Design review of the part built by this model. Coordinates are the model's own, in mm. Round coordinates to 2 decimals unless told otherwise and drop trailing zeros. Loops run counter-clockwise (first coordinate to the right, second up) from the corner with the lowest first, then second, coordinate; pieces in that order, holes last. Notation, with made-up numbers: M 55.5,-40 L 110.5,-40 A16 ccw 110.5,-21 Z; hole C -37,41.5 d1. An arc over 180 degrees is marked long. Use a Markdown table: item, result.
from build123d import *

# Parameters (mm, degrees)
ESQUISSE1_W              = 160
ESQUISSE1_H              = 210
BOSS_EXTRU_1_DEPTH       = 3
CONG_6_R                 = 2
ESQUISSE4_R              = 1.5
ENL_V_MAT_EXTRU_3_DEPTH  = 4
ESQUISSE6_W              = 45
ESQUISSE6_H              = 70
ENL_V_MAT_EXTRU_5_DEPTH  = 4
ESQUISSE7_R              = 15
ENL_V_MAT_EXTRU_6_DEPTH  = 856
ESQUISSE8_R              = 15
ENL_V_MAT_EXTRU_7_DEPTH  = 856
ESQUISSE9_R              = 7.5
ENL_V_MAT_EXTRU_8_DEPTH  = 856
ESQUISSE10_R             = 7.5
ENL_V_MAT_EXTRU_13_DEPTH = 856
ESQUISSE12_W             = 30
ESQUISSE12_H             = 15
ENL_V_MAT_EXTRU_14_DEPTH = 856
ESQUISSE13_W             = 160
ESQUISSE13_H             = 3
BOSS_EXTRU_2_DEPTH       = 3
ESQUISSE14_W             = 3
ESQUISSE14_H             = 213
BOSS_EXTRU_3_DEPTH       = 3
ESQUISSE15_W             = 3
ESQUISSE15_H             = 70
ENL_V_MAT_EXTRU_15_DEPTH = 4
ESQUISSE18_W             = 3
ESQUISSE18_H             = 213
BOSS_EXTRU_4_DEPTH       = 3
ESQUISSE19_W             = 166
ESQUISSE19_H             = 3
BOSS_EXTRU_5_DEPTH       = 3
ESQUISSE20_W             = 3
ESQUISSE20_H             = 70
ENL_V_MAT_EXTRU_16_DEPTH = 3
ESQUISSE21_R             = 1.5
ENL_V_MAT_EXTRU_17_DEPTH = 3
ESQUISSE22_R             = 1.5
ENL_V_MAT_EXTRU_18_DEPTH = 3
ESQUISSE23_R             = 1.5
ENL_V_MAT_EXTRU_19_DEPTH = 3
CONG_7_R                 = 2
CONG_8_R                 = 2
CONG_9_R                 = 2


with BuildPart() as part:
    # Esquisse1 → Boss.-Extru.1 (new body)
    with BuildSketch(Plane.XY):
        with Locations((-86.269341233, 25.410958904)):
            Rectangle(ESQUISSE1_W, ESQUISSE1_H)
    extrude(amount=BOSS_EXTRU_1_DEPTH)

    # Congé6
    cong_6_edges = [part.edges().sort_by_distance(p)[0] for p in [
        (-166.269341233, 130.410958904, 1.5),
    ]]
    fillet(cong_6_edges, radius=CONG_6_R)

    # Esquisse4 → Enlèv. mat.-Extru.3 (cut)
    with BuildSketch(Plane.XY.offset(3)):
        with Locations((-164.469341233, 128.610958904)):
            Circle(ESQUISSE4_R)
    extrude(amount=-ENL_V_MAT_EXTRU_3_DEPTH, mode=Mode.SUBTRACT)

    # Esquisse6 → Enlèv. mat.-Extru.5 (cut)
    with BuildSketch(Plane.XY.offset(3)):
        with Locations((-28.769341233, -31.589041096)):
            Rectangle(ESQUISSE6_W, ESQUISSE6_H)
    extrude(amount=-ENL_V_MAT_EXTRU_5_DEPTH, mode=Mode.SUBTRACT)

    # Esquisse7 → Enlèv. mat.-Extru.6 (cut)
    with BuildSketch(Plane.XY.offset(3)):
        with Locations((-101.269341233, -47.589041096)):
            Circle(ESQUISSE7_R)
    extrude(amount=-ENL_V_MAT_EXTRU_6_DEPTH, mode=Mode.SUBTRACT)

    # Esquisse8 → Enlèv. mat.-Extru.7 (cut)
    with BuildSketch(Plane.XY.offset(3)):
        with Locations((-143.966076441, -9.589041096)):
            Circle(ESQUISSE8_R)
    extrude(amount=-ENL_V_MAT_EXTRU_7_DEPTH, mode=Mode.SUBTRACT)

    # Esquisse9 → Enlèv. mat.-Extru.8 (cut)
    with BuildSketch(Plane.XY.offset(3)):
        with Locations((-139.269341233, -44.589041096)):
            Circle(ESQUISSE9_R)
    extrude(amount=-ENL_V_MAT_EXTRU_8_DEPTH, mode=Mode.SUBTRACT)

    # Esquisse10 → Enlèv. mat.-Extru.13 (cut)
    with BuildSketch(Plane.XY.offset(3)):
        with Locations((-158.469341233, -44.589041096)):
            Circle(ESQUISSE10_R)
    extrude(amount=-ENL_V_MAT_EXTRU_13_DEPTH, mode=Mode.SUBTRACT)

    # Esquisse12 → Enlèv. mat.-Extru.14 (cut)
    with BuildSketch(Plane.XY.offset(3)):
        with Locations((-61.269341233, 122.910958904)):
            Rectangle(ESQUISSE12_W, ESQUISSE12_H)
    extrude(amount=-ENL_V_MAT_EXTRU_14_DEPTH, mode=Mode.SUBTRACT)

    # Esquisse13 → Boss.-Extru.2 (add)
    with BuildSketch(Plane.XZ.offset(79.589041096)):
        with Locations((-86.269341233, 1.5)):
            Rectangle(ESQUISSE13_W, ESQUISSE13_H)
    extrude(amount=BOSS_EXTRU_2_DEPTH)

    # Esquisse14 → Boss.-Extru.3 (add)
    with BuildSketch(Plane(origin=(-6.269341233, 0, 0), x_dir=(0, 0, -1), z_dir=(1, 0, 0))):
        with Locations((-1.5, 23.910958904)):
            Rectangle(ESQUISSE14_W, ESQUISSE14_H)
    extrude(amount=BOSS_EXTRU_3_DEPTH)

    # Esquisse15 → Enlèv. mat.-Extru.15 (cut)
    with BuildSketch(Plane(origin=(-3.269341233, 0, 0), x_dir=(0, 0, -1), z_dir=(1, 0, 0))):
        with Locations((-1.5, -31.589041096)):
            Rectangle(ESQUISSE15_W, ESQUISSE15_H)
    extrude(amount=-ENL_V_MAT_EXTRU_15_DEPTH, mode=Mode.SUBTRACT)

    # Esquisse18 → Boss.-Extru.4 (add)
    with BuildSketch(Plane(origin=(-3.269341233, 0, 0), x_dir=(0, 0, -1), z_dir=(1, 0, 0))):
        with Locations((-1.5, 23.910958904)):
            Rectangle(ESQUISSE18_W, ESQUISSE18_H)
    extrude(amount=BOSS_EXTRU_4_DEPTH)

    # Esquisse19 → Boss.-Extru.5 (add)
    with BuildSketch(Plane(origin=(0, -82.589041096, 0), x_dir=(-1, 0, 0), z_dir=(0, -1, 0))):
        with Locations((83.269341233, -1.5)):
            Rectangle(ESQUISSE19_W, ESQUISSE19_H)
    extrude(amount=BOSS_EXTRU_5_DEPTH)

    # Esquisse20 → Enlèv. mat.-Extru.16 (cut)
    with BuildSketch(Plane(origin=(-0.269341233, 0, 0), x_dir=(0, 0, -1), z_dir=(1, 0, 0))):
        with Locations((-1.5, -31.589041096)):
            Rectangle(ESQUISSE20_W, ESQUISSE20_H)
    extrude(amount=-ENL_V_MAT_EXTRU_16_DEPTH, mode=Mode.SUBTRACT)

    # Esquisse21 → Enlèv. mat.-Extru.17 (cut)
    with BuildSketch(Plane.XY.offset(3)):
        with Locations((-2.069341233, 128.610958904)):
            Circle(ESQUISSE21_R)
    extrude(amount=-ENL_V_MAT_EXTRU_17_DEPTH, mode=Mode.SUBTRACT)

    # Esquisse22 → Enlèv. mat.-Extru.18 (cut)
    with BuildSketch(Plane.XY.offset(3)):
        with Locations((-2.069341233, -83.789041096)):
            Circle(ESQUISSE22_R)
    extrude(amount=-ENL_V_MAT_EXTRU_18_DEPTH, mode=Mode.SUBTRACT)

    # Esquisse23 → Enlèv. mat.-Extru.19 (cut)
    with BuildSketch(Plane.XY.offset(3)):
        with Locations((-164.469341233, -83.789041096)):
            Circle(ESQUISSE23_R)
    extrude(amount=-ENL_V_MAT_EXTRU_19_DEPTH, mode=Mode.SUBTRACT)

    # Congé7
    cong_7_edges = [part.edges().sort_by_distance(p)[0] for p in [
        (-0.269341233, -85.589041096, 1.5),
    ]]
    fillet(cong_7_edges, radius=CONG_7_R)

    # Congé8
    cong_8_edges = [part.edges().sort_by_distance(p)[0] for p in [
        (-0.269341233, 130.410958904, 1.5),
    ]]
    fillet(cong_8_edges, radius=CONG_8_R)

    # Congé9
    cong_9_edges = [part.edges().sort_by_distance(p)[0] for p in [
        (-166.269341233, -85.589041096, 1.5),
    ]]
    fillet(cong_9_edges, radius=CONG_9_R)


solid = part.part
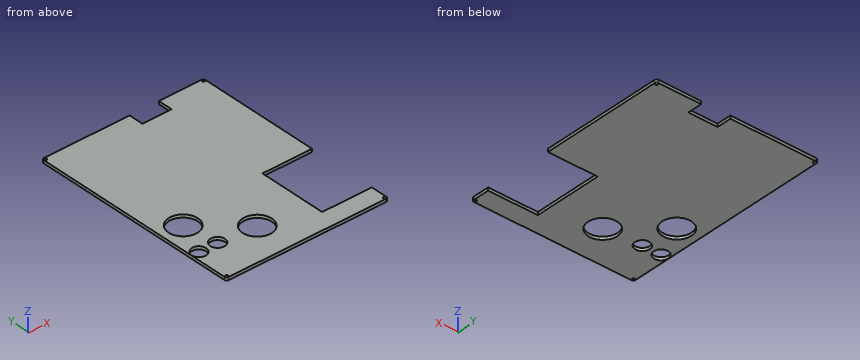
1. Take a section at C-C on z = 1.3. Count the separate pieces of the cut face and the enclosed holes in it, and give its area (3 significant figures).
Check values:
| item | result |
|---|---|
| separate pieces | 1 |
| enclosed holes | 8 |
| area | 30,000 mm² |
2. Wall thickness on line 1 along Y through (x, z) = (-18, 0.2); line 2 along X through (y, z) = (-10, 2); line 3 along X through (y, z) = (-13, 0.25): over which ranges is each line inside the solid? List them lowest first. Write a range as from..to.
Check values:
| item | result |
|---|---|
| line 1 | y = -85.59..-66.59, 3.41..130.41 |
| line 2 | x = -166.27..-158.96, -128.97..-51.27 |
| line 3 | x = -166.27..-158.57, -129.36..-51.27 |
3. Insertion check: pin 1 (1.5 mm diameter, centred on x = -64.5, z = 1.5, fed in from +Y); pin 2 (0.9 mm diameter, centred on y = -25, z = 1, fed in from +X). Each pin has a flat end and moves straight along its axis. Give the tip position at first contact, or say it passes through.
Check values:
| item | result |
|---|---|
| pin 1 | stops at y = 115.41 |
| pin 2 | stops at x = -51.27 |
4. Take a section at D-D on x = -54. Give the boundary of the cut face in (y, z).
Check values:
| item | result |
|---|---|
| outline | M -85.59,0 L 115.41,0 L 115.41,3 L -85.59,3 Z |
5. Take a section at B-B on y = -20.5. Give the boundary of the cut face in (x, z).
Check values:
| item | result |
|---|---|
| outline | M -166.27,0 L -154.26,0 L -154.26,3 L -166.27,3 Z; M -133.67,0 L -51.27,0 L -51.27,3 L -133.67,3 Z |
6. Take a section at A-A on x = -17.5. Give the boundary of the cut face in (y, z).
Check values:
| item | result |
|---|---|
| outline | M -85.59,0 L -66.59,0 L -66.59,3 L -85.59,3 Z; M 3.41,0 L 130.41,0 L 130.41,3 L 3.41,3 Z |
